from build123d import *

# Parameters (mm, degrees)
BOSS_EXTRUDE1_DEPTH = 40
SKETCH2_W           = 34
SKETCH2_H           = 34
CUT_EXTRUDE1_DEPTH  = 448.413276673
FILLET1_R           = 1


with BuildPart() as part:
    # Sketch1 → Boss-Extrude1 (new body)
    with BuildSketch(Plane.XY):
        Polygon((0, 0), (-441.284874285, 62.018544574), (-435.717950246, 101.629267323), (0, 40.393102901), align=None)
    extrude(amount=BOSS_EXTRUDE1_DEPTH)

    # Sketch2 → Cut-Extrude1 (cut, through all)
    with BuildSketch(Plane(origin=(-441.284874285, 62.018544574, 0), x_dir=(0, 0, 1), z_dir=(-0.9902680687415704, 0.13917310096006613, 0))):
        with Locations((20, 20)):
            Rectangle(SKETCH2_W, SKETCH2_H)
    extrude(amount=-CUT_EXTRUDE1_DEPTH, mode=Mode.SUBTRACT)

    # Fillet1
    fillet1_edges = [part.edges().sort_by_distance(p)[0] for p in [
        (-438.501412265, 81.823905948, 40),
        (-220.642437142, 31.009272287, 40),
        (0, 20.19655145, 40),
        (-220.642437142, 31.009272287, 0),
        (-438.501412265, 81.823905948, 0),
        (-217.858975123, 71.011185112, 0),
        (0, 20.19655145, 0),
        (-217.858975123, 71.011185112, 40),
        (0, 0, 20),
        (-441.284874285, 62.018544574, 20),
        (-435.717950246, 101.629267323, 20),
        (0, 40.393102901, 20),
    ]]
    fillet(fillet1_edges, radius=FILLET1_R)


solid = part.part
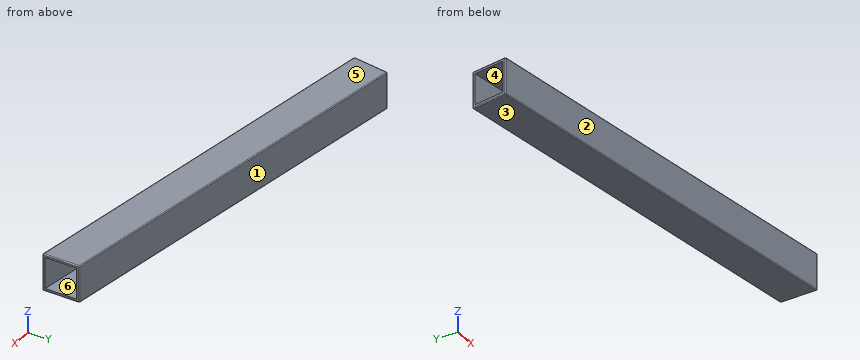
For this review, take the finished solid that the model builds, in its own axes (mm). Face numbers are marked on the shaded views. A direction names the side the tool comes from. Give positions to 0.01 mm unless a question says otherwise; leave off trailing zeros. Order: outer loops, then holes, each group sorted by start corner. A loop starts at its lowest first (then second) coordinate and runs counter-clockwise, first axis right, second up. Notation, with made-up numbers: M 10.5,71.25 L 67.5,71.25 A14 ccw 67.5,97.25 Z; hole C 2,40 d11. An arc over 180 degrees is marked long. Answer in a Markdown table with one row per item. Add a question column.
(1) For the marked faces 5 and 6, list the 3-axis set-ups (+Z, -Z, +X, -X, +Y, -Y) from which the entire face can be reached by the end or side of a thin tool; tool diameter is ignored.
(2) Wall thickness on probe 1 along Z at (x, y) = (-332.5, 74.5); probe 2 along Y at (x, z) = (-270, 12.5); probe 3 along Y at (x, z) = (-155, 16): over which ranges is each line inside the solid? List them lowest first. Write a range as [from, to].
(3) Mouldability with a two-part tool opening along Y and no side actions: class the marked faces 1, 2, 3 and 4 as +Y half, -Y half, draft (parallel to the pull), parting line (faces both ways), or undercut.
(4) Consider section A-A on z = 31.5. State the section outline as (x, y) points, and give its area (3 significant figures).
(5) For pin 1 (6 mm diameter, centred on y = 74, z = 34.5, fed in from -X); pin 2 (6 mm diameter, centred on x = -234.5, z = 6.5, fed in from +Y); pin 3 (2 mm diameter, centred on x = -102.5, z = 15, fed in from -Y), all flat-tipped, find the tip position at first contact; note any pin that passes through.
Evaluation:
| question | item | result |
|---|---|---|
| 1 | face 5 | +Z, +X, -X, +Y, -Y |
| 1 | face 6 | none |
| 2 | probe 1 | z = [0, 3], [37, 40] |
| 2 | probe 2 | y = [37.95, 40.98], [75.31, 78.34] |
| 2 | probe 3 | y = [21.78, 24.81], [59.15, 62.18] |
| 3 | face 1 | +Y half |
| 3 | face 2 | -Y half |
| 3 | face 3 | draft |
| 3 | face 4 | undercut |
| 4 | outline | M -441.15,63.01 A1 ccw -440.29,61.88 L -1.14,0.16 A1 ccw 0,1.15 L 0,3.03 L -440.87,64.99 Z; M -436.14,98.66 L 0,37.36 L 0,39.52 A1 ccw -0.86,40.51 L -434.73,101.49 A1 ccw -435.86,100.64 Z |
| 4 | area | 2,660 mm^2 |
| 5 | pin 1 | stops at x = -439.83 |
| 5 | pin 2 | stops at y = 73.77 |
| 5 | pin 3 | stops at y = 14.26 |
